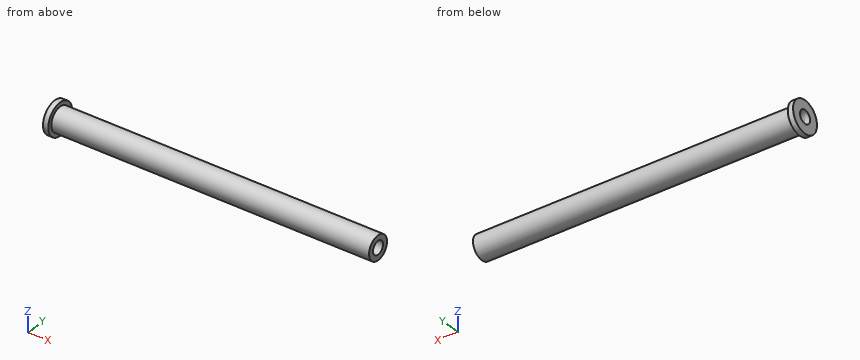
Solid Edge part; units mm, degrees
sketch "Sketch1" plane through (0, 0, 0) normal (1, 0, 0) x (0, 1, 0)
  circle A0 centre (0, 0) radius 4.5
  circle A1 centre (0, 0) radius 2.5
extrude "Protrusion1" add sketch "Sketch1" along normal mid plane 120
sketch "Sketch2" plane through (-60, 0, 0) normal (-1, 0, 0) x (0, 0, 1)
  circle A0 centre (0, 0) radius 2.5
  circle A1 centre (0, 0) radius 6
extrude "Wyciągnięcie_2" add sketch "Sketch2" along normal blind 2
Model file for the job. Use its own axes, mm. Round coordinates to 2 decimals unless told otherwise and drop trailing zeros. Loops run counter-clockwise (first coordinate to the right, second up) from the corner with the lowest first, then second, coordinate; pieces in that order, holes last. Notation, with made-up numbers: (62.25, 1.25) -> (66.25, 1.25) arc R28 ccw to (66.25, 28.25) -> close; hole circle Ø3 at (19.25, 36). An arc over 180 degrees is marked (long way). Answer as CSV lines item,"result". Start each with the question number.
1) Slice it at C-C (x = 30.5). List the corners of the cut face in (y, z).
2) Slice it at A-A (z = 0). List the corners of the cut face in (x, y), plus the area to 3 significant figures.
3) Probe line 1 along Z through (x, y) = (-29.5, 0); line 2 along Y through (x, z) = (2, 3.75); line 3 along X through (y, z) = (2.5, 4.5). List the from-to ranges inside material, lowest first.
4) Pin check, flat tips, straight feed: P1, Ø6.5, axis at y = 0, z = 0, coming from the +X side; P2, Ø4, axis at x = 39.5, y = -1, coming from the +Z side; P3, Ø4, axis at y = 0, z = 0, coming from the -X side; P4, Ø2, axis at x = 6.5, y = 3.5, coming from the -Z side. Stop position of each tip, or through.
Filled in:
1,outline,"circle Ø9 at (0, 0); hole circle Ø5 at (0, 0)"
2,outline,"(-62, -6) -> (-60, -6) -> (-60, -4.5) -> (60, -4.5) -> (60, -2.5) -> (-62, -2.5) -> close; (-62, 2.5) -> (60, 2.5) -> (60, 4.5) -> (-60, 4.5) -> (-60, 6) -> (-62, 6) -> close"
2,area,"494 mm2"
3,line 1,"z = -4.5 to -2.5, 2.5 to 4.5"
3,line 2,"y = -2.49 to 2.49"
3,line 3,"x = -62 to -60"
4,P1,"stops at x = 60"
4,P2,"stops at z = 4.5"
4,P3,"passes through"
4,P4,"stops at z = -3.74"
